Build history of the part. All positions in model axes, mm. Face numbers are marked on the shaded views. A direction names the side the tool comes from. Round coordinates to 2 decimals unless told otherwise and drop trailing zeros. Write each loop counter-clockwise with the first axis right and the second up, starting at its lowest first coordinate (ties: lowest second). Pieces come first, ordered by that corner, then holes. Notation, with made-up numbers: (-12.5, 85.5) -> (14.5, 85.5) arc R22 cw to (14.5, 116.5) -> close; hole circle Ø6 at (3.5, 31.25). An arc over 180 degrees is marked (long way). Return JSON: item names as keys, results as strings.
from build123d import *

# Parameters (mm, degrees)
CYLINDER007_R     = 1.25
CYLINDER007_DEPTH = 10
CYLINDER029_W     = 4
CYLINDER029_H     = 26
CYLINDER029_ANGLE = 180
BOX006_W          = 29
BOX006_H          = 2.75
BOX006_DEPTH      = 2


with BuildPart() as b_no:
    # Cylinder007 → Cylinder007 (new body)
    with BuildSketch(Plane(origin=(57, -1, 4), x_dir=(1, 0, 0), z_dir=(0, 0, 1))):
        Circle(CYLINDER007_R)
    extrude(amount=CYLINDER007_DEPTH)


with BuildPart() as s016:
    # Cylinder029 → Cylinder029 (revolve)
    with BuildSketch(Plane(origin=(57, 0, -14), x_dir=(-1, 0, 0), z_dir=(0, 1, 0))):
        with Locations((2, 13)):
            Rectangle(CYLINDER029_W, CYLINDER029_H)
    revolve(axis=Axis((57, 0, -14), (0, 0, 1)), revolution_arc=CYLINDER029_ANGLE)


with BuildPart() as obj1:
    # Box006 → Box006 (new body)
    with BuildSketch(Plane(origin=(42, 0, 10), x_dir=(1, 0, 0), z_dir=(0, 0, 1))):
        with Locations((14.5, 1.375)):
            Rectangle(BOX006_W, BOX006_H)
    extrude(amount=BOX006_DEPTH)

    # Fusion008: union S016
    add(s016.part)

    # Cut014: cut B_NO
    add(b_no.part, mode=Mode.SUBTRACT)


with BuildPart() as obj1_1:
    # Cut014 placement: moved
    add(obj1.part.moved(Location((-1, 0, 0))))


solid = obj1_1.part
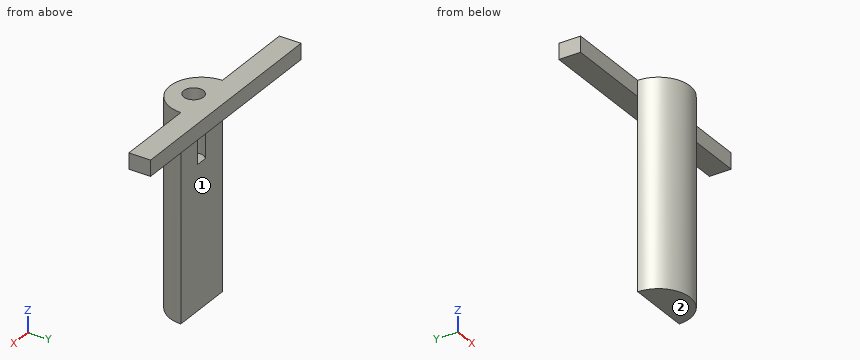
Q1. Saw through at A-A on x = 56. List the corners of the cut face in (y, z), then the cut area to 3 significant figures.
Verdict:
{"outline": "(-4, -14) -> (0, -14) -> (0, 4) -> (-2.25, 4) -> (-2.25, 12) -> (-4, 12) -> close; (0.25, 10) -> (2.75, 10) -> (2.75, 12) -> (0.25, 12) -> close", "area": "91.0 mm²"}
Q2. Saw through at D-D on x = 64.5. List the corners of the cut face in (y, z), then the cut area to 3 significant figures.
Verdict:
{"outline": "(0, 10) -> (2.75, 10) -> (2.75, 12) -> (0, 12) -> close", "area": "5.50 mm²"}
Q3. Saw through at B-B on z = 8.5. List the corners of the cut face in (x, y), then the cut area to 3 significant figures.
Verdict:
{"outline": "(52, 0) arc R4 ccw to (60, 0) -> (56.75, 0) arc R1.25 cw (long way) to (55.25, 0) -> close", "area": "20.5 mm²"}
Q4. 3-axis set-ups, long thin cutter, end or side, ignore diameter. For the marked faces 1 and 2: which of +Z, -Z, +X, -X, +Y, -Y reach the whole face in a straight line?
Verdict:
{"face 1": "-Z, +X, -X, +Y", "face 2": "-Z, +X, -X, +Y, -Y"}
Q5. Pin check, flat tips, straight feed: pin 1 Ø2.5 at (x, z) = (57.5, 3.5) entering from +Y; pin 2 Ø0.6 at (x, z) = (44, 11) entering from -Y; pin 3 Ø2 at (y, z) = (-0.5, -9) entering from +X. Stop position of each tip, or through.
Verdict:
{"pin 1": "stops at y = 0", "pin 2": "stops at y = 0", "pin 3": "stops at x = 60"}
Q6. Saw through at C-C on y = -1.5. List the corners of the cut face in (x, z).
Verdict:
{"outline": "(52.29, -14) -> (59.71, -14) -> (59.71, 12) -> (57.15, 12) -> (57.15, 4) -> (54.85, 4) -> (54.85, 12) -> (52.29, 12) -> close"}
Q7. Wall check: L1, parallel to Y at x = 56, z = 6; L2, parallel to Z at x = 62.75, y = 2; L3, parallel to X at y = -1, z = 10.75. Give the ranges that are in metal, low to high.
Verdict:
{"L1": "y = -4 to -2.25", "L2": "z = 10 to 12", "L3": "x = 52.13 to 54.75, 57.25 to 59.87"}
